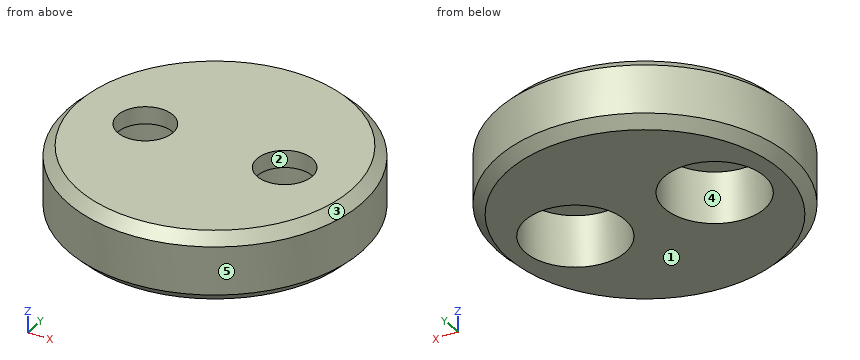
from build123d import *

# Parameters (mm, degrees)
ESQUISSE1_R             = 8.5
ESQUISSE1_R_2           = 1.6
BOSS_EXTRU_1_DEPTH      = 4
ESQUISSE3_R             = 2.9
ENL_V_MAT_EXTRU_1_DEPTH = 3
CHANFREIN1_SIZE         = 0.6


with BuildPart() as part:
    # Esquisse1 → Boss.-Extru.1 (new body)
    with BuildSketch(Plane.XY):
        Circle(ESQUISSE1_R)
        with Locations((-4, 0)):
            Circle(ESQUISSE1_R_2, mode=Mode.SUBTRACT)
        with Locations((4, 0)):
            Circle(ESQUISSE1_R_2, mode=Mode.SUBTRACT)
    extrude(amount=BOSS_EXTRU_1_DEPTH)

    # Esquisse3 → Enlèv. mat.-Extru.1 (cut)
    with BuildSketch(Plane(origin=(0, 0, 0), x_dir=(-1, 0, 0), z_dir=(0, 0, -1))):
        with Locations((4, 0)):
            Circle(ESQUISSE3_R)
        with Locations((-4, 0)):
            Circle(ESQUISSE3_R)
    extrude(amount=-ENL_V_MAT_EXTRU_1_DEPTH, mode=Mode.SUBTRACT)

    # Chanfrein1
    chanfrein1_edges = [part.edges().sort_by_distance(p)[0] for p in [
        (-8.5, 0, 0),
        (-8.5, 0, 4),
    ]]
    chamfer(chanfrein1_edges, length=CHANFREIN1_SIZE)


solid = part.part
For this review, take the finished solid that the model builds, in its own axes (mm). Face numbers are marked on the shaded views. A direction names the side the tool comes from. Coordinates: 2 decimals unless noted, no trailing zeros. Loops run counter-clockwise (first coordinate to the right, second up) from the corner with the lowest first, then second, coordinate; pieces in that order, holes last. Notation, with made-up numbers: (-33.5, 32.5) - (-29.5, 32.5) arc R21 ccw to (-29.5, 37.5) - close; hole circle Ø4 at (51, 75.5). An arc over 180 degrees is marked (long way). Use a Markdown table: item, result. Add a question column.
Item 1: For line 1 (X direction, y = -0.25, z = 2.5); line 2 (X direction, y = 1, z = 2.65); line 3 (Z direction, x = -3, y = 2.5), list the stretches that pass through material, from the lowest coordinate up.
Item 2: We need section B-B (z = 1.65). Give the boundary of the cut face in (x, y), and give its area (3 significant figures).
Item 3: Tool access review of the marked faces 4 and 5: name each direction out of +Z, -Z, +X, -X, +Y, -Y from which nothing blocks a thin tool from reaching the whole face with its end or side.
Item 4: Insertion check: pin 1 Ø1 at (x, z) = (2.5, 1.5) entering from -Y; pin 2 Ø4.5 at (x, y) = (4, 0) entering from -Z; pin 3 Ø2.5 at (x, y) = (-4, 0) entering from +Z; pin 4 Ø1.5 at (y, z) = (-6.5, 3.5) entering from -X. Each pin has a flat end and moves straight along its axis. Give the tip position at first contact, or say it passes through.
Item 5: We need section A-A (y = 0). Give the boundary of the cut face in (x, z).
Item 6: Mouldability with a two-part tool opening along Y and no side actions: class the marked faces 1, 2 and 3 as pulls with the +Y half, pulls with the -Y half, needs draft (parallel to the pull), parting line crosses it, or undercut.
Item 7: We need section C-C (z = 3.6). Give the boundary of the cut face in (x, y), and give its area (3 significant figures).
Results list:
| question | item | result |
|---|---|---|
| 1 | line 1 | x = -8.5 to -6.89, -1.11 to 1.11, 6.89 to 8.5 |
| 1 | line 2 | x = -8.44 to -6.72, -1.28 to 1.28, 6.72 to 8.44 |
| 1 | line 3 | z = 3 to 4 |
| 2 | outline | circle Ø17 at (0, 0); hole circle Ø5.8 at (-4, 0); hole circle Ø5.8 at (4, 0) |
| 2 | area | 174 mm^2 |
| 3 | face 4 | -Z |
| 3 | face 5 | +Z, -Z |
| 4 | pin 1 | stops at y = -8.26 |
| 4 | pin 2 | stops at z = 3 |
| 4 | pin 3 | passes through |
| 4 | pin 4 | stops at x = -6.25 |
| 5 | outline | (-8.5, 0.6) - (-7.9, 0) - (-6.9, 0) - (-6.9, 3) - (-5.6, 3) - (-5.6, 4) - (-7.9, 4) - (-8.5, 3.4) - close; (-2.4, 3) - (-1.1, 3) - (-1.1, 0) - (1.1, 0) - (1.1, 3) - (2.4, 3) - (2.4, 4) - (-2.4, 4) - close; (5.6, 3) - (6.9, 3) - (6.9, 0) - (7.9, 0) - (8.5, 0.6) - (8.5, 3.4) - (7.9, 4) - (5.6, 4) - close |
| 6 | face 1 | needs draft |
| 6 | face 2 | undercut |
| 6 | face 3 | parting line crosses it |
| 7 | outline | circle Ø16.6 at (0, 0); hole circle Ø3.2 at (-4, 0); hole circle Ø3.2 at (4, 0) |
| 7 | area | 200 mm^2 |
